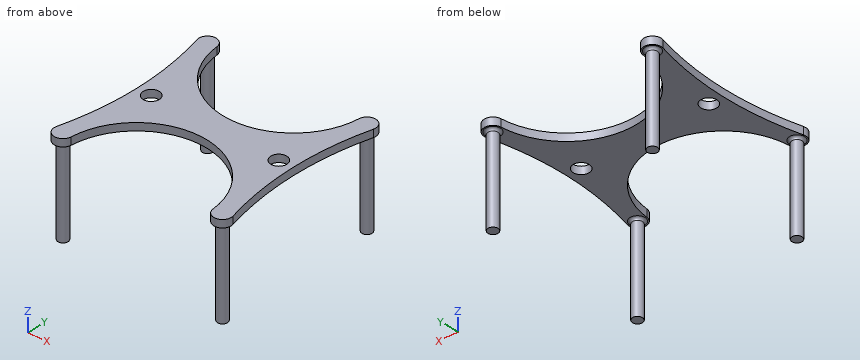
from build123d import *

# Parameters (mm, degrees)
SKETCH_R     = 3.2
PAD_DEPTH    = 3
SKETCH001_R  = 2
PAD001_DEPTH = 35.2
FILLET_R     = 1


with BuildPart() as part:
    # Sketch → Pad (new body)
    with BuildSketch(Plane.XY):
        with BuildLine():
            ThreePointArc((-28.263319, 32.055045), (0, 6.156485), (28.263319, 32.055045))
            ThreePointArc((35.13074, 30.844133), (32.357769, 35.196827), (28.263319, 32.055045))
            ThreePointArc((35.13074, 30.844133), (31.070033, 0), (35.13074, -30.844133))
            ThreePointArc((28.263319, -32.055045), (32.357769, -35.196827), (35.13074, -30.844133))
            ThreePointArc((28.263319, -32.055045), (0, -6.156485), (-28.263319, -32.055045))
            ThreePointArc((-35.13074, -30.844133), (-32.357769, -35.196827), (-28.263319, -32.055045))
            ThreePointArc((-35.13074, -30.844133), (-31.070033, 0), (-35.13074, 30.844133))
            ThreePointArc((-28.263319, 32.055045), (-32.357769, 35.196827), (-35.13074, 30.844133))
        make_face()
        with Locations((-25.4, 0)):
            Circle(SKETCH_R, mode=Mode.SUBTRACT)
        with Locations((25.4, 0)):
            Circle(SKETCH_R, mode=Mode.SUBTRACT)
    extrude(amount=PAD_DEPTH)

    # Sketch001 → Pad001 (join)
    with BuildSketch(Plane(origin=(0, 0, 0), x_dir=(1, 0, 0), z_dir=(0, 0, -1))):
        with Locations((-31.75, 31.75)):
            Circle(SKETCH001_R)
        with Locations((31.75, 31.75)):
            Circle(SKETCH001_R)
        with Locations((-31.75, -31.75)):
            Circle(SKETCH001_R)
        with Locations((31.75, -31.75)):
            Circle(SKETCH001_R)
    extrude(amount=PAD001_DEPTH)

    # Fillet
    fillet_edges = [part.edges().sort_by_distance(p)[0] for p in [
        (29.75, 31.75, 0),
        (29.75, -31.75, 0),
        (-33.75, 31.75, 0),
        (-33.75, -31.75, 0),
    ]]
    fillet(fillet_edges, radius=FILLET_R)


solid = part.part
Design review of the part built by this model. Coordinates are the model's own, in mm. Coordinates: 2 decimals unless noted, no trailing zeros. Order: outer loops, then holes, each group sorted by start corner. A loop starts at its lowest first (then second) coordinate and runs counter-clockwise, first axis right, second up.
Item 1: Take a section at A-A, the plane y = 0. Write out the cut boundary in (x, z).
Item 2: Take a section at C-C, the plane x = -25.4. Write out the cut boundary in (y, z).
Item 3: For line 1 (X direction, y = 31.5, z = -8); line 2 (Z direction, x = 25, y = -16.5); line 3 (Y direction, x = 25.4, z = 2.15), list the stretches that pass through material, from the lowest coordinate up.
Item 4: Take a section at B-B, the plane y = 26.5. Write out the cut boundary in (x, z).
Item 5: Take a section at D-D, the plane z = -22.5. Write out the cut boundary in (x, y).
Item 6: For pin 1 Ø12 at (x, y) = (12.5, 19.5) entering from +Z; pin 2 Ø4 at (x, y) = (-23, 11) entering from -Z; pin 3 Ø12 at (y, z) = (-26, -11.5) entering from +X, all flat-tipped, find the tip position at first contact; note any pin that passes through.
The answers:
1. outline: (-31.07, 0) - (-28.6, 0) - (-28.6, 3) - (-31.07, 3) - close; (-22.2, 0) - (22.2, 0) - (22.2, 3) - (-22.2, 3) - close; (28.6, 0) - (31.07, 0) - (31.07, 3) - (28.6, 3) - close
2. outline: (-21.89, 0) - (-3.2, 0) - (-3.2, 3) - (-21.89, 3) - close; (3.2, 0) - (21.89, 0) - (21.89, 3) - (3.2, 3) - close
3. line 1: x = -33.73 to -29.77, 29.77 to 33.73
3. line 2: z = 0 to 3
3. line 3: y = -21.89 to -3.2, 3.2 to 21.89
4. outline: (-34.05, 0) - (-27.21, 0) - (-27.21, 3) - (-34.05, 3) - close; (27.21, 0) - (34.05, 0) - (34.05, 3) - (27.21, 3) - close
5. outline: circle Ø4 at (-31.75, -31.75); circle Ø4 at (-31.75, 31.75); circle Ø4 at (31.75, -31.75); circle Ø4 at (31.75, 31.75)
6. pin 1: passes through
6. pin 2: stops at z = 0
6. pin 3: stops at x = 33.75
